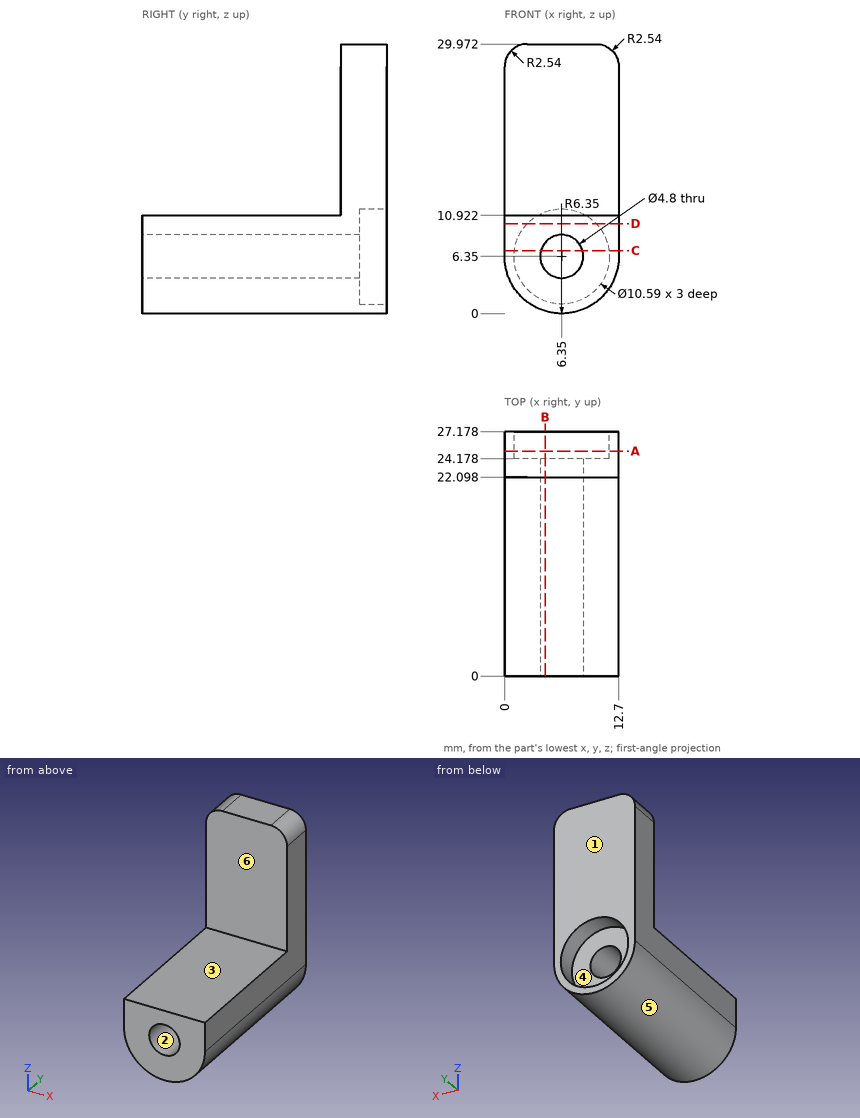
Geometry: see drawing. Coordinates: mm, zero at the bounding-box minimum. A direction names the side the tool comes from. Give positions to 0.01 mm unless a question says otherwise; leave off trailing zeros. Loops run counter-clockwise (first coordinate to the right, second up) from the corner with the lowest first, then second, coordinate; pieces in that order, holes last. Notation, with made-up numbers: (-27.75, -31) -> (4.25, -31) arc R24 ccw to (4.25, -5) -> close; hole circle Ø9 at (-28.5, 84). An arc over 180 degrees is marked (long way). Put each result on its own line as item: value.
1. Cut plane B-B (x = 4.5). Return the cut outline in (y, z), plus the area to 3 significant figures.
Taken from the geometry:
outline: (0, 0.28) -> (27.18, 0.28) -> (27.18, 1.39) -> (24.18, 1.39) -> (24.18, 4.82) -> (0, 4.82) -> close; (0, 7.88) -> (24.18, 7.88) -> (24.18, 11.31) -> (27.18, 11.31) -> (27.18, 29.97) -> (22.1, 29.97) -> (22.1, 10.92) -> (0, 10.92) -> close
area: 282 mm2
2. Pin query (flat end, axial travel): P1, Ø3, axis at x = 2, y = 23.5, coming from the -Z side; P2, Ø6.5, axis at x = 7, y = 16.5, coming from the +Z side; P3, Ø1.5, axis at x = 4.5, y = 17.5, coming from the -Z side; P4, Ø6, axis at x = 2, z = 7.5, coming from the +Y side. Return the tip coordinate at first contact, or that it passes through.
Taken from the geometry:
P1: stops at z = 0.68
P2: stops at z = 10.92
P3: stops at z = 0.1
P4: stops at y = 27.18
3. Cut plane D-D (z = 10). Return the cut outline in (x, y).
Taken from the geometry:
outline: (0, 0) -> (12.7, 0) -> (12.7, 27.18) -> (10.19, 27.18) -> (10.19, 24.18) -> (2.51, 24.18) -> (2.51, 27.18) -> (0, 27.18) -> close
4. Set-up query: the marked faces 4, 5 and 6. Return all of +Z, -Z, +X, -X, +Y, -Y with unobstructed straight access to the full face (end or side cutting, diameter ignored); none if empty.
Taken from the geometry:
face 4: +Y
face 5: -Z, +Y, -Y
face 6: +Z, +X, -X, -Y
5. Cut plane A-A (y = 25). Return the cut outline in (x, z) (3 decimals).
Taken from the geometry:
outline: (0, 6.35) arc R6.35 ccw to (12.7, 6.35) -> (12.7, 27.432) arc R2.54 ccw to (10.16, 29.972) -> (2.54, 29.972) arc R2.54 ccw to (0, 27.432) -> close; hole circle Ø10.59 at (6.35, 6.35)
6. Ray query, line 1 along Z through (x, y) = (6.35, 16); line 2 along Z through (x, y) = (6.35, 26.1) (3 decimals); line 3 along Y through (x, z) = (3.5, 18.5). Return the intervals inside material, ascending. Write a range as [from, to].
Taken from the geometry:
line 1: z = [0, 3.95], [8.75, 10.92]
line 2: z = [0, 1.055], [11.645, 29.972]
line 3: y = [22.1, 27.18]
7. Pull-direction query (Z, two-part tool) for the marked faces 1, 2 and 3; classes: released by +Z, released by -Z, zero draft, split by the parting line, or undercut.
Taken from the geometry:
face 1: zero draft
face 2: undercut
face 3: released by +Z
8. Cut plane C-C (z = 7). Return the cut outline in (x, y), plus the area to 3 significant figures.
Taken from the geometry:
outline: (0, 0) -> (4.04, 0) -> (4.04, 24.18) -> (1.1, 24.18) -> (1.1, 27.18) -> (0, 27.18) -> close; (8.66, 0) -> (12.7, 0) -> (12.7, 27.18) -> (11.6, 27.18) -> (11.6, 24.18) -> (8.66, 24.18) -> close
area: 202 mm2
